Verification items for the finished model (mm, model axes). A direction names the side the tool comes from. Give positions to 0.01 mm unless a question says otherwise; leave off trailing zeros. Write each loop counter-clockwise with the first axis right and the second up, starting at its lowest first coordinate (ties: lowest second). Pieces come first, ordered by that corner, then holes. Notation, with made-up numbers: (11.25, 34) -> (66.25, 34) arc R18 cw to (66.25, 64) -> close; hole circle Ø5 at (19, -18.75). An arc over 180 degrees is marked (long way). Use one line per item in the form item = value. Start each with the question number.
(1) Section check B-B, the plane y = -13.5. Record the cut outline in (x, z).
(2) Section check C-C, the plane x = 38. Record the cut outline in (y, z).
(3) Set-up check for faces 1 (the face through (10, -27, 532)), 2 (the face through (36, -57, 532)), 3 (the face through (0, -14, 532)): record each of +Z, -Z, +X, -X, +Y, -Y from which the full face is reachable in a straight line by a thin tool's end or side.
(4) Depth check by flat-ended pin: pin 1 Ø22 at (x, z) = (10, 312.5) entering from -Y; pin 2 Ø4 at (y, z) = (-15, 609.5) entering from +X; pin 3 Ø6 at (y, z) = (-44, 522.5) entering from +X; pin 4 Ø10 at (y, z) = (-43.5, 340.5) entering from -X. Enter the tip coordinate at first touch or a pass-through.
(5) Section check A-A, the plane z = 834. Record the cut outline in (x, y).
(6) Scan lines: L1, parallel to Y at x = 17.5, z = 679.5; L2, parallel to Y at x = 20.5, z = 344.5; L3, parallel to X at y = -52, z = 962. Record each from-to range of solid material in increasing order.
from build123d import *

# Parameters (mm, degrees)
CROQUIS1_W              = 6
CROQUIS1_H              = 1050
SALIENTE_EXTRUIR1_DEPTH = 23
CROQUIS2_W              = 24
CROQUIS2_H              = 4
SALIENTE_EXTRUIR2_DEPTH = 1050
CROQUIS3_W              = 4
CROQUIS3_H              = 30
SALIENTE_EXTRUIR3_DEPTH = 1050
CROQUIS4_W              = 29
CROQUIS4_H              = 4
SALIENTE_EXTRUIR4_DEPTH = 1050


with BuildPart() as part:
    # Croquis1 → Saliente-Extruir1 (new body)
    with BuildSketch(Plane(origin=(0, 0, 0), x_dir=(1, 0, 0), z_dir=(0, 1, 0))):
        with Locations((3, -525)):
            Rectangle(CROQUIS1_W, CROQUIS1_H)
    extrude(amount=-SALIENTE_EXTRUIR1_DEPTH)

    # Croquis2 → Saliente-Extruir2 (add)
    with BuildSketch(Plane.XY.offset(1050)):
        with Locations((12, -25)):
            Rectangle(CROQUIS2_W, CROQUIS2_H)
    extrude(amount=-SALIENTE_EXTRUIR2_DEPTH)

    # Croquis3 → Saliente-Extruir3 (add)
    with BuildSketch(Plane.XY.offset(1050)):
        with Locations((22, -42)):
            Rectangle(CROQUIS3_W, CROQUIS3_H)
    extrude(amount=-SALIENTE_EXTRUIR3_DEPTH)

    # Croquis4 → Saliente-Extruir4 (add)
    with BuildSketch(Plane.XY.offset(1050)):
        with Locations((34.5, -59)):
            Rectangle(CROQUIS4_W, CROQUIS4_H)
    extrude(amount=-SALIENTE_EXTRUIR4_DEPTH)


solid = part.part
Completed:
q1.outline = (0, 0) -> (6, 0) -> (6, 1050) -> (0, 1050) -> close
q2.outline = (-61, 0) -> (-57, 0) -> (-57, 1050) -> (-61, 1050) -> close
q3.face_1 = +Z, -Z, -X, -Y
q3.face_2 = +Z, -Z, +X, +Y
q3.face_3 = +Z, -Z, -X, +Y, -Y
q4.pin_1 = -61
q4.pin_2 = 6
q4.pin_3 = 24
q4.pin_4 = 20
q5.outline = (0, -27) -> (20, -27) -> (20, -61) -> (49, -61) -> (49, -57) -> (24, -57) -> (24, -23) -> (6, -23) -> (6, 0) -> (0, 0) -> close
q6.L1 = -27 to -23
q6.L2 = -61 to -23
q6.L3 = 20 to 24
